Autodesk Inventor part; units mm, degrees
ref_plane "YZ Plane" through (0, 0, 0) normal (1, 0, 0) x (0, 1, 0)
ref_plane "XZ Plane" through (0, 0, 0) normal (0, 1, 0) x (-1, 0, 0)
ref_plane "XY Plane" through (0, 0, 0) normal (0, 0, 1) x (1, 0, 0)
sketch "Sketch1" plane through (0, 0, 0) normal (0, 0, 1) x (1, 0, 0)
  line L0 (0, 0) -> (-672.6812, 0)
  line L1 (-672.6812, 0) -> (-672.6812, -1000)
  line L2 (-672.6812, -1000) -> (0, -1000)
  line L3 (0, -1000) -> (0, 0)
extrude "Extrusion1" add sketch "Sketch1" along normal blind 6
sketch "Sketch2" plane through (0, 0, 6) normal (0, 0, 1) x (1, 0, 0)
  line L0 (-50, -800) -> (-305, -800)
  line L1 (-305, -800) -> (-305, -950)
  line L2 (-305, -950) -> (-50, -950)
  line L3 (-50, -950) -> (-50, -800)
  line L4 (-672.6812, -1000) -> (0, -1000)
  point P0 (0, 0)
  dimension "d2" = 150
  dimension "d3" = 255
  dimension "d4" = 50
  dimension "d5" = 50
extrude "Extrusion2" cut sketch "Sketch2" against normal through all
properties part number "capot"
Model file for the job. Use its own axes, mm. Coordinates: 2 decimals unless noted, no trailing zeros. Order: outer loops, then holes, each group sorted by start corner. A loop starts at its lowest first (then second) coordinate and runs counter-clockwise, first axis right, second up. Notation, with made-up numbers: M 12,87 L 41,87 A15 cw 41,106 Z; hole C 36.25,7 d11. An arc over 180 degrees is marked long. Return JSON: item names as keys, results as strings.
1. Saw through at B-B (z = 1.35). Give the cut face in (x, y), and give its area (3 significant figures).
Ans:
{"outline": "M -672.68,-1000 L 0,-1000 L 0,0 L -672.68,0 Z; hole M -305,-950 L -50,-950 L -50,-800 L -305,-800 Z", "area": "634,000 mm^2"}
2. Drill centre lines: probe 1 along Y at (x, z) = (-268, 1.05); probe 2 along X at (y, z) = (-836.5, 4.05). Where is each one in solid material? Low to high.
Ans:
{"probe 1": "-1000 to -950, -800 to 0", "probe 2": "-672.68 to -305, -50 to 0"}
3. Saw through at A-A (x = -101.5). Give the cut face in (y, z).
Ans:
{"outline": "M -1000,0 L -950,0 L -950,6 L -1000,6 Z; M -800,0 L 0,0 L 0,6 L -800,6 Z"}
4. Flat gauge pin, fed straight in: pin 1 (1.5 mm diameter, centred on x = -450, z = 1, fed in from +Y). Where does the tip first touch, or does it go through?
Ans:
{"pin 1": "y = 0"}
